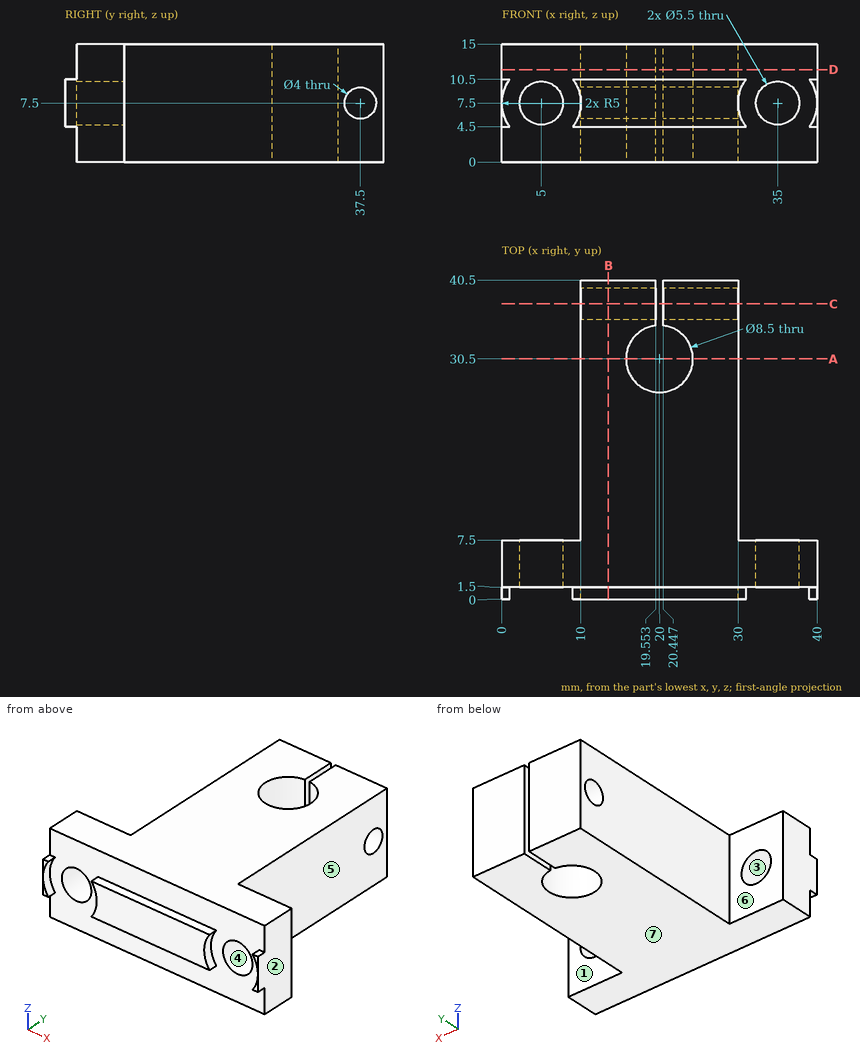
The drawing under review shows one solid part. Ordinate dimensions are in mm from its lowest x, y, z. A direction names the side the tool comes from. Coordinates: 2 decimals unless noted, no trailing zeros. Loops run counter-clockwise (first coordinate to the right, second up) from the corner with the lowest first, then second, coordinate; pieces in that order, holes last. Notation, with made-up numbers: (33, 57.25) -> (62, 57.25) arc R23 cw to (62, 69.25) -> close; hole circle Ø6 at (-20.75, -36). An arc over 180 degrees is marked (long way). Answer as a JSON object with one key per item and string values.
Q1. Tool access review of the marked faces 5, 6 and 7: name each direction out of +Z, -Z, +X, -X, +Y, -Y from which nothing blocks a thin tool from reaching the whole face with its end or side.
Answer block:
{"face 5": "+Z, -Z, +X, +Y", "face 6": "+Z, -Z, -X, +Y", "face 7": "-Z, +X, -X, +Y, -Y"}
Q2. Take a section at B-B on x = 13.5. Give the boundary of the cut face in (y, z).
Answer block:
{"outline": "(0, 4.5) -> (1.5, 4.5) -> (1.5, 0) -> (40.5, 0) -> (40.5, 15) -> (1.5, 15) -> (1.5, 10.5) -> (0, 10.5) -> close; hole circle Ø4 at (37.5, 7.5)"}
Q3. Take a section at D-D on z = 11.75. Give the boundary of the cut face in (x, y), plus the area to 3 significant figures.
Answer block:
{"outline": "(0, 1.5) -> (40, 1.5) -> (40, 7.5) -> (30, 7.5) -> (30, 40.5) -> (20.45, 40.5) -> (20.45, 34.73) arc R4.25 cw (long way) to (19.55, 34.73) -> (19.55, 40.5) -> (10, 40.5) -> (10, 7.5) -> (0, 7.5) -> close", "area": "838 mm^2"}
Q4. Clearance check with flat-ended pins moving along their axes: pin 1 Ø4.5 at (y, z) = (38.5, 4) entering from +X; pin 2 Ø2.5 at (y, z) = (37.5, 7.5) entering from +X; pin 3 Ø3 at (y, z) = (38.5, 10) entering from -X; pin 4 Ø0.8 at (x, y) = (39.5, 1) entering from -Z. State where each tip first meets the part, or that it passes through.
Answer block:
{"pin 1": "stops at x = 30", "pin 2": "passes through", "pin 3": "stops at x = 10", "pin 4": "stops at z = 4.5"}
Q5. To check wall thickness, follow L1, parallel to X at y = 4.95, z = 7.5; L2, parallel to X at y = 6.5, z = 6 (1 decimal); L3, parallel to Y at x = 14, z = 7.5. State the ranges of each line that lie inside material, in increasing order.
Answer block:
{"L1": "x = 0 to 2.25, 7.75 to 32.25, 37.75 to 40", "L2": "x = 0 to 2.7, 7.3 to 32.7, 37.3 to 40", "L3": "y = 0 to 35.5, 39.5 to 40.5"}
Q6. The part is to be moulded in two halves that separate along X. For the marked faces 1, 2, 3 and 4, say which applies: +X half, -X half, draft (parallel to the pull), parting line (faces both ways), or undercut.
Answer block:
{"face 1": "draft", "face 2": "+X half", "face 3": "undercut", "face 4": "undercut"}
Q7. Take a section at C-C on y = 37.5. Give the boundary of the cut face in (x, z).
Answer block:
{"outline": "(10, 0) -> (19.55, 0) -> (19.55, 5.5) -> (10, 5.5) -> close; (10, 9.5) -> (19.55, 9.5) -> (19.55, 15) -> (10, 15) -> close; (20.45, 0) -> (30, 0) -> (30, 5.5) -> (20.45, 5.5) -> close; (20.45, 9.5) -> (30, 9.5) -> (30, 15) -> (20.45, 15) -> close"}
Q8. Take a section at A-A on y = 30.5. Give the boundary of the cut face in (x, z).
Answer block:
{"outline": "(10, 0) -> (15.75, 0) -> (15.75, 15) -> (10, 15) -> close; (24.25, 0) -> (30, 0) -> (30, 15) -> (24.25, 15) -> close"}
